Model file for the job. Use its own axes, mm. Face numbers are marked on the shaded views. A direction names the side the tool comes from. Round coordinates to 2 decimals unless told otherwise and drop trailing zeros. Order: outer loops, then holes, each group sorted by start corner. A loop starts at its lowest first (then second) coordinate and runs counter-clockwise, first axis right, second up. Notation, with made-up numbers: (25, -37.5) - (73, -37.5) arc R16 cw to (73, -27.5) - close; hole circle Ø3 at (-25.75, -23). An arc over 180 degrees is marked (long way). Answer as CSV lines item,"result". Start each with the question number.
1. Wall check: line 1 along Z through (x, y) = (-0.25, 3.75); line 2 along Z through (x, y) = (1.75, 0); line 3 along Y through (x, z) = (-0.75, 15.5). Give the ranges that are in metal, low to high. Write a range as [from, to].
2. Band-saw the part on A-A on z = 1.5. List the corners of the cut face in (x, y), then the cut area to 3 significant figures.
3. Band-saw the part on C-C on z = 9.5. List the corners of the cut face in (x, y), then the cut area to 3 significant figures.
4. Band-saw the part on B-B on y = 0. List the corners of the cut face in (x, z), then the cut area to 3 significant figures.
5. 3-axis set-ups, long thin cutter, end or side, ignore diameter. For the marked faces 5 and 6: which of +Z, -Z, +X, -X, +Y, -Y reach the whole face in a straight line?
6. Pull direction X, two halves, no side cores. Call the marked faces 1, 2, 3 and 4: released by +X, released by -X, zero draft, split by the parting line, or undercut.
7. Pin check, flat tips, straight feed: pin 1 Ø3 at (y, z) = (-2, 10.5) entering from +X; pin 2 Ø4 at (y, z) = (3, 12) entering from +X; pin 3 Ø4 at (y, z) = (2, 10.5) entering from -X. Stop position of each tip, or through.
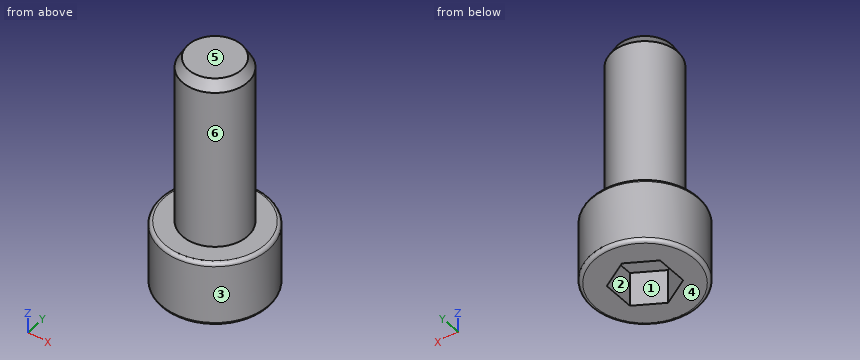
```python
from build123d import *

# Parameters (mm, degrees)
CUT_EXTRUDE1_DEPTH  = 2.54
SKETCH3_R           = 2.413
BOSS_EXTRUDE1_DEPTH = 12.7
CHAMFER1_SIZE       = 0.762
CHAMFER1_SIZE2      = 0.439940905


with BuildPart() as part:
    # Sketch1 → Revolve1 (revolve)
    with BuildSketch(Plane(origin=(0, 0, 0), x_dir=(1, 0, 0), z_dir=(0, 1, 0))):
        with BuildLine():
            Line((0, 0), (3.71475, 0))
            ThreePointArc((3.71475, 0), (3.894355122, -0.074394878), (3.96875, -0.254))
            Line((3.96875, -0.254), (3.96875, -4.572))
            ThreePointArc((3.96875, -4.572), (3.894355122, -4.751605122), (3.71475, -4.826))
            Line((3.71475, -4.826), (0, -4.826))
            Line((0, -4.826), (0, 0))
        make_face()
    revolve(axis=Axis((0, 0, 0), (0, 0, -1)))

    # Sketch2 → Cut-Extrude1 (cut)
    with BuildSketch(Plane(origin=(0, 0, 0), x_dir=(-1, 0, 0), z_dir=(0, 0, -1))):
        Polygon((0, 2.291358881), (-1.984375, 1.14567944), (-1.984375, -1.14567944), (0, -2.291358881), (1.984375, -1.14567944), (1.984375, 1.14567944), align=None)
    extrude(amount=-CUT_EXTRUDE1_DEPTH, mode=Mode.SUBTRACT)

    # Sketch3 → Boss-Extrude1 (add)
    with BuildSketch(Plane.XY.offset(4.826)):
        Circle(SKETCH3_R)
    extrude(amount=BOSS_EXTRUDE1_DEPTH)

    # Chamfer1
    chamfer1_edges = [part.edges().sort_by_distance(p)[0] for p in [
        (-2.413, 0, 17.526),
    ]]
    chamfer1_side = [part.faces().sort_by_distance(p)[0] for p in [
        (-2.413, 0, 11.176),
    ]]
    chamfer(chamfer1_edges, length=CHAMFER1_SIZE, length2=CHAMFER1_SIZE2, reference=chamfer1_side[0])


solid = part.part
```
Reply:
1,line 1,"z = [0, 4.82]"
1,line 2,"z = [2.54, 17.53]"
1,line 3,"y = [-2.29, 2.29]"
2,outline,"circle Ø7.94 at (0, 0); hole (-1.98, -1.15) - (0, -2.29) - (1.98, -1.15) - (1.98, 1.15) - (0, 2.29) - (-1.98, 1.15) - close"
2,area,"35.8 mm2"
3,outline,"circle Ø4.83 at (0, 0)"
3,area,"18.3 mm2"
4,outline,"(-3.97, 0.25) arc R0.25 ccw to (-3.71, 0) - (-1.98, 0) - (-1.98, 2.54) - (1.98, 2.54) - (1.98, 0) - (3.71, 0) arc R0.25 ccw to (3.97, 0.25) - (3.97, 4.57) arc R0.25 ccw to (3.71, 4.83) - (2.41, 4.83) - (2.41, 16.76) - (1.97, 17.53) - (-1.97, 17.53) - (-2.41, 16.76) - (-2.41, 4.83) - (-3.71, 4.83) arc R0.25 ccw to (-3.97, 4.57) - close"
4,area,"89.1 mm2"
5,face 5,"+Z, +X, -X, +Y, -Y"
5,face 6,"+Z"
6,face 1,"undercut"
6,face 2,"undercut"
6,face 3,"split by the parting line"
6,face 4,"zero draft"
7,pin 1,"stops at x = 2.36"
7,pin 2,"stops at x = 2.2"
7,pin 3,"stops at x = -2.41"
